```python
from build123d import *

# Parameters (mm, degrees)
SKETCH1_R           = 1.25
BOSS_EXTRUDE1_DEPTH = 3


with BuildPart() as part:
    # Sketch1 → Boss-Extrude1 (new body)
    with BuildSketch(Plane.XY):
        with BuildLine():
            Line((-42.5, -27.5), (-42.5, -25))
            Line((-42.5, -25), (42.5, -25))
            Line((42.5, -25), (42.5, -27.5))
            ThreePointArc((42.5, -27.5), (46.5, -31.5), (50.5, -27.5))
            Line((50.5, -27.5), (50.5, -25))
            Line((50.5, -25), (50.5, 25))
            Line((50.5, 25), (50.5, 27.5))
            ThreePointArc((50.5, 27.5), (46.5, 31.5), (42.5, 27.5))
            Line((42.5, 27.5), (42.5, 25))
            Line((42.5, 25), (-42.5, 25))
            Line((-42.5, 25), (-42.5, 27.5))
            ThreePointArc((-42.5, 27.5), (-46.5, 31.5), (-50.5, 27.5))
            Line((-50.5, 27.5), (-50.5, 25))
            Line((-50.5, 25), (-50.5, -25))
            Line((-50.5, -25), (-50.5, -27.5))
            ThreePointArc((-50.5, -27.5), (-46.5, -31.5), (-42.5, -27.5))
        make_face()
        with Locations((-46.5, 27.5)):
            Circle(SKETCH1_R, mode=Mode.SUBTRACT)
        with Locations((46.5, 27.5)):
            Circle(SKETCH1_R, mode=Mode.SUBTRACT)
        with Locations((46.5, -27.5)):
            Circle(SKETCH1_R, mode=Mode.SUBTRACT)
        with Locations((-46.5, -27.5)):
            Circle(SKETCH1_R, mode=Mode.SUBTRACT)
    extrude(amount=BOSS_EXTRUDE1_DEPTH)


solid = part.part
```
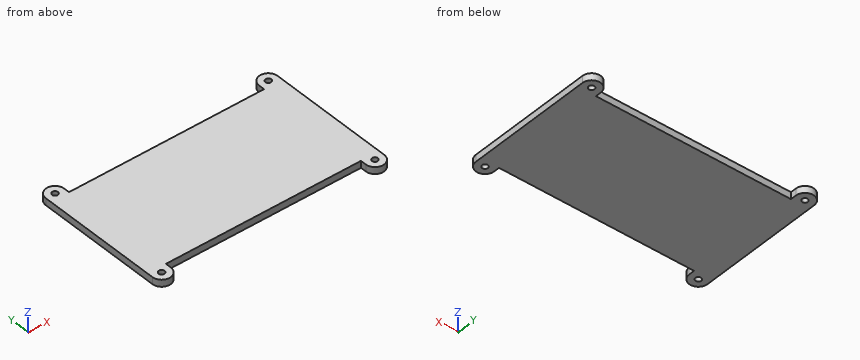
Model file for the job. Use its own axes, mm. Round coordinates to 2 decimals unless told otherwise and drop trailing zeros. Write each loop counter-clockwise with the first axis right and the second up, starting at its lowest first coordinate (ties: lowest second). Pieces come first, ordered by that corner, then holes. Notation, with made-up numbers: M -12,40 L -1,40 A23 cw -1,59 Z; hole C 73.5,35.25 d6. An arc over 180 degrees is marked long. Put each result on its own line as item: value.
Item 1: Cut at B-B (z = 2.55). List the corners of the cut face in (x, y).
Responses:
outline: M -50.5,-27.5 A4 ccw -42.5,-27.5 L -42.5,-25 L 42.5,-25 L 42.5,-27.5 A4 ccw 50.5,-27.5 L 50.5,27.5 A4 ccw 42.5,27.5 L 42.5,25 L -42.5,25 L -42.5,27.5 A4 ccw -50.5,27.5 Z; hole C -46.5,-27.5 d2.5; hole C -46.5,27.5 d2.5; hole C 46.5,-27.5 d2.5; hole C 46.5,27.5 d2.5
Item 2: Probe L1, parallel to Y at x = -46.5, z = 1.45; L2, parallel to X at y = -26, z = 0.6; L3, parallel to X at y = 28.5, z = 2.3. List the from-to ranges inside material, lowest first. Write a range as from..to.
Responses:
L1: -31.5..-28.75, -26.25..26.25, 28.75..31.5
L2: -50.5..-42.5, 42.5..50.5
L3: -50.37..-47.25, -45.75..-42.63, 42.63..45.75, 47.25..50.37
Item 3: Flat gauge pin, fed straight in: P1, Ø1.5, axis at x = 10, z = 1, coming from the -Y side. Where does the tip first touch, or does it go through?
Responses:
P1: y = -25
Item 4: Cut at A-A (x = 46.5). List the corners of the cut face in (y, z), and give its area (3 significant figures).
Responses:
outline: M -31.5,0 L -28.75,0 L -28.75,3 L -31.5,3 Z; M -26.25,0 L 26.25,0 L 26.25,3 L -26.25,3 Z; M 28.75,0 L 31.5,0 L 31.5,3 L 28.75,3 Z
area: 174 mm²
